Can you work these out from the model? Positions are in its coordinate system, mm. Round coordinates to 2 decimals unless told otherwise and drop trailing zeros. Order: outer loops, then holes, each group sorted by start corner. A loop starts at its lowest first (then second) coordinate and runs counter-clockwise, first axis right, second up. Notation, with made-up numbers: (-2.5, 30) -> (54.5, 30) arc R18 ccw to (54.5, 63) -> close; hole circle Ø11 at (-17.75, 40). An arc over 180 degrees is marked (long way). Use a Markdown table: item, result. Add a question column.
Q1. I'm going to push flat-ended pins straight in: pin 1 Ø20.5 at (x, y) = (-17.78, 34.036) entering from +Z; pin 2 Ø14 at (x, y) = (18.034, 34.036) entering from -Z. Where does each tip first touch, or does it pass through?
Q2. I need wall thicknesses on line 1 along Y through (x, z) = (17.5, -0.2); line 2 along X through (y, z) = (39, -0.2); line 3 along X through (y, z) = (40, -0.05). Which ranges of each line are inside material? Lowest first, please. Write a range as [from, to].
Q3. If we section it at C-C on z = -0.2: List the corners of the cut face in (x, y) for me, plus the area to 3 significant figures.
Q4. If we section it at A-A on x = -17.78: List the corners of the cut face in (y, z) for me.
Q5. If we section it at B-B on y = -6: List the corners of the cut face in (x, z) for me, plus the area to 3 significant figures.
```python
from build123d import *

# Parameters (mm, degrees)
BOSS_EXTRUDE1_DEPTH = 0.254
SKETCH2_R           = 7.874
CUT_EXTRUDE1_DEPTH  = 0.254
SKETCH3_R           = 16.002
CUT_EXTRUDE2_DEPTH  = 0.254


with BuildPart() as part:
    # Sketch1 → Boss-Extrude1 (new body)
    with BuildSketch(Plane.XY):
        with BuildLine():
            Line((-27.94, -44.196), (27.94, -44.196))
            ThreePointArc((27.94, -44.196), (30.813681959, -43.005681959), (32.004, -40.132))
            Line((32.004, -40.132), (32.004, 40.132))
            ThreePointArc((32.004, 40.132), (30.813681959, 43.005681959), (27.94, 44.196))
            Line((27.94, 44.196), (-27.94, 44.196))
            ThreePointArc((-27.94, 44.196), (-30.813681959, 43.005681959), (-32.004, 40.132))
            Line((-32.004, 40.132), (-32.004, -40.132))
            ThreePointArc((-32.004, -40.132), (-30.813681959, -43.005681959), (-27.94, -44.196))
        make_face()
    extrude(amount=-BOSS_EXTRUDE1_DEPTH)

    # Sketch2 → Cut-Extrude1 (cut)
    with BuildSketch(Plane.XY):
        with Locations((18.034, 34.036)):
            Circle(SKETCH2_R)
        with Locations((-17.78, 34.036)):
            Circle(SKETCH2_R)
    extrude(amount=-CUT_EXTRUDE1_DEPTH, mode=Mode.SUBTRACT)

    # Sketch3 → Cut-Extrude2 (cut)
    with BuildSketch(Plane.XY):
        with Locations((0.508, 0.254)):
            Circle(SKETCH3_R)
    extrude(amount=-CUT_EXTRUDE2_DEPTH, mode=Mode.SUBTRACT)


solid = part.part
```
Answer below:
| question | item | result |
|---|---|---|
| 1 | pin 1 | z = 0 |
| 1 | pin 2 | through |
| 2 | line 1 | [-44.2, 26.18], [41.89, 44.2] |
| 2 | line 2 | [-32, -23.89], [-11.67, 11.92], [24.15, 32] |
| 2 | line 3 | [-32, -22.92], [-12.64, 12.89], [23.18, 32] |
| 3 | outline | (-32, -40.13) arc R4.06 ccw to (-27.94, -44.2) -> (27.94, -44.2) arc R4.06 ccw to (32, -40.13) -> (32, 40.13) arc R4.06 ccw to (27.94, 44.2) -> (-27.94, 44.2) arc R4.06 ccw to (-32, 40.13) -> close; hole circle Ø15.75 at (-17.78, 34.04); hole circle Ø32 at (0.51, 0.25); hole circle Ø15.75 at (18.03, 34.04) |
| 3 | area | 4,450 mm² |
| 4 | outline | (-44.2, -0.25) -> (26.16, -0.25) -> (26.16, 0) -> (-44.2, 0) -> close; (41.91, -0.25) -> (44.2, -0.25) -> (44.2, 0) -> (41.91, 0) -> close |
| 5 | outline | (-32, -0.25) -> (-14.22, -0.25) -> (-14.22, 0) -> (-32, 0) -> close; (15.24, -0.25) -> (32, -0.25) -> (32, 0) -> (15.24, 0) -> close |
| 5 | area | 8.78 mm² |
